Job drawing, mm, ordinate dimensions from the low corner. One solid piece. Give positions to 0.01 mm unless a question says otherwise; leave off trailing zeros. Order: outer loops, then holes, each group sorted by start corner. A loop starts at its lowest first (then second) coordinate and runs counter-clockwise, first axis right, second up. Notation, with made-up numbers: M -22.75,35.5 L 23.25,35.5 A8 ccw 23.25,41.5 Z; hole C 80,-29 d8. An arc over 180 degrees is marked long. One line per item, written item: value. Start each with the question number.
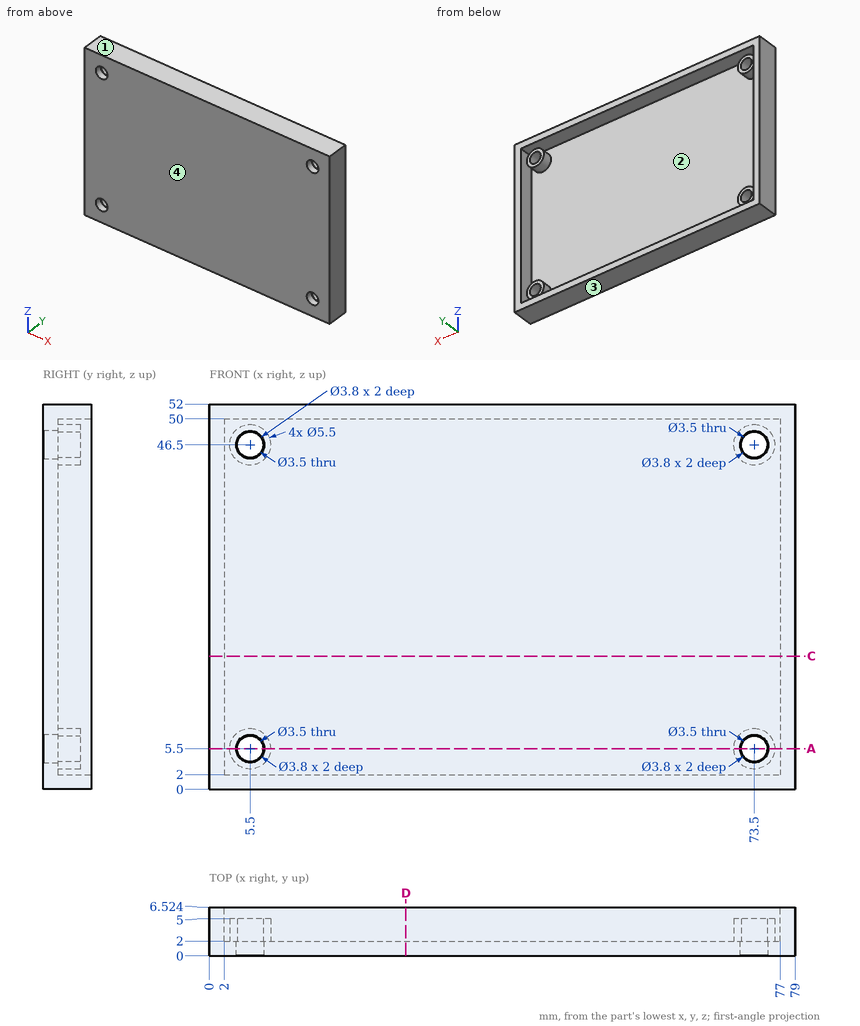
1) Slice it at D-D (x = 26.5). List the corners of the cut face in (y, z), plus the area to 3 significant figures.
2) Pull direction Z, two halves, no side cores. Call the marked faces 1, 2, 3 and 4: pulls with the +Z half, pulls with the -Z half, needs draft (parallel to the pull), parting line crosses it, or undercut.
3) Drop flat-ended pins along their axis: P1, Ø3, axis at x = 72.5, z = 4.5, coming from the +Y side; P2, Ø3, axis at x = 60.5, z = 25, coming from the +Y side. Give the stop position or say it passes through.
4) Drill centre lines: line 1 (X direction, y = 2.9, z = 46.5); line 2 (X direction, y = 1.55, z = 46.5); line 3 (Z direction, x = 73.5, y = 1.55). Where is each one in solid material? Low to high.
5) Slice it at A-A (z = 5.5). State how many separate pieces and enclosed holes the cut face has, plus the area to 3 significant figures.
6) Slice it at C-C (z = 18). List the corners of the cut face in (x, y).
Results list:
1. outline: M 0,0 L 6.52,0 L 6.52,2 L 2,2 L 2,50 L 6.52,50 L 6.52,52 L 0,52 Z
1. area: 122 mm²
2. face 1: pulls with the +Z half
2. face 2: undercut
2. face 3: pulls with the -Z half
2. face 4: needs draft
3. P1: stops at y = 5
3. P2: stops at y = 2
4. line 1: x = 0 to 2, 2.75 to 3.75, 7.25 to 8.25, 70.75 to 71.75, 75.25 to 76.25, 77 to 79
4. line 2: x = 0 to 3.6, 7.4 to 71.6, 75.4 to 79
4. line 3: z = 0 to 3.6, 7.4 to 44.6, 48.4 to 52
5. separate pieces: 3
5. enclosed holes: 0
5. area: 173 mm²
6. outline: M 0,0 L 79,0 L 79,6.52 L 77,6.52 L 77,2 L 2,2 L 2,6.52 L 0,6.52 Z
